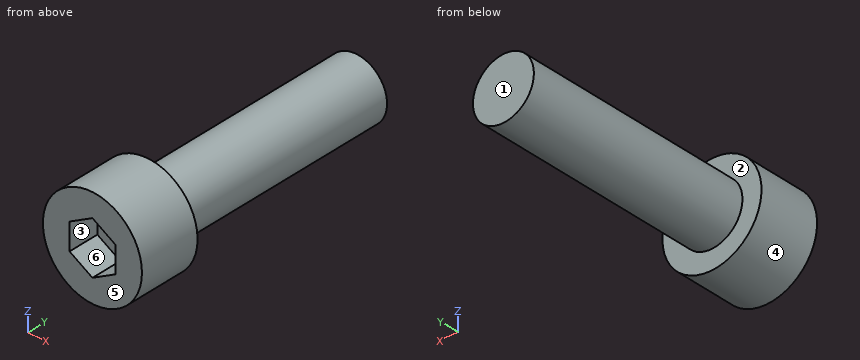
Solid Edge part; units mm, degrees
sketch "Sketch1" plane through (0, 0, 0) normal (0, -1, 0) x (1, 0, 0)
  circle A0 centre (0, 0) radius 6.5
extrude "Protrusion1" add sketch "Sketch1" against normal blind 8
sketch "Sketch2" plane through (0, 0, 0) normal (0, -1, 0) x (1, 0, 0)
  line L0 (3, 1.7321) -> (0, 3.4641)
  line L1 (0, 3.4641) -> (-3, 1.7321)
  line L2 (-3, 1.7321) -> (-3, -1.7321)
  line L3 (-3, -1.7321) -> (0, -3.4641)
  line L4 (0, -3.4641) -> (3, -1.7321)
  line L5 (3, -1.7321) -> (3, 1.7321)
extrude "ExtrudedCutout_1" cut sketch "Sketch2" against normal blind 4
sketch "Sketch3" plane through (0, 8, 0) normal (0, 1, 0) x (-1, 0, 0)
  circle A0 centre (0, 0) radius 4
extrude "ExtrudedProtrusion_2" add sketch "Sketch3" along normal blind 30
cosmetic_thread "Thread1"
properties material "Steel"
Could you check a few things on this model? Use its own coordinates, in mm. Face numbers are marked on the shaded views. A direction names the side the tool comes from. Coordinates: 2 decimals unless noted, no trailing zeros. Order: outer loops, then holes, each group sorted by start corner. A loop starts at its lowest first (then second) coordinate and runs counter-clockwise, first axis right, second up. Notation, with made-up numbers: (-16, -18) - (26, -18) arc R6 ccw to (26, -10) - close; hole circle Ø11 at (-18, 67). An arc over 180 degrees is marked (long way). Answer in a Markdown table with one row per item. Add a question column.
(1) If we section it at C-C, the plane y = 13: Please give me the cut outline in (x, z), then the cut area to 3 significant figures.
(2) If we section it at D-D, the plane z = 5.5: Please give me the cut outline in (x, y).
(3) I need wall thicknesses on L1, parallel to Y at x = -4, z = -3; L2, parallel to X at y = 18, z = -0.25; L3, parallel to Y at x = 2, z = -1.25. Which ranges of each line are inside material? Lowest first, please.
(4) If we section it at A-A, the plane z = 0: Please give me the cut outline in (x, y).
(5) Will these pins go through, and if not, where does the flat tip stop? pin 1 (4 mm diameter, centred on x = -1, y = 8.5, fed in from +Z); pin 2 (2 mm diameter, centred on x = 1.5, z = -1, fed in from -Y); pin 3 (1 mm diameter, centred on y = 20.5, z = 0, fed in from +X); pin 4 (6 mm diameter, centred on x = -3, y = 32.5, fed in from -Z).
(6) On a 3-axis mill with a long thin cutter (end or side, diameter ignored), from which of +Z, -Z, +X, -X, +Y, -Y can I reach the whole of each face in a straight line? I mean the marked faces 1, 2 and 3. Say none if no direction works.
(7) If we mould it in two halves opening along Z, with no side actions, what happens to the marked faces 4, 5 and 6? For each: released by +Z, released by -Z, zero draft, split by the parting line, or undercut.
(8) If we section it at B-B, the plane x = -1.25: Please give me the cut outline in (y, z), then the cut area to 3 significant figures.
Results are:
| question | item | result |
|---|---|---|
| 1 | outline | circle Ø8 at (0, 0) |
| 1 | area | 50.3 mm2 |
| 2 | outline | (-3.46, 0) - (3.46, 0) - (3.46, 8) - (-3.46, 8) - close |
| 3 | L1 | y = 0 to 8 |
| 3 | L2 | x = -3.99 to 3.99 |
| 3 | L3 | y = 4 to 38 |
| 4 | outline | (-6.5, 0) - (-3, 0) - (-3, 4) - (3, 4) - (3, 0) - (6.5, 0) - (6.5, 8) - (4, 8) - (4, 38) - (-4, 38) - (-4, 8) - (-6.5, 8) - close |
| 5 | pin 1 | stops at z = 6.5 |
| 5 | pin 2 | stops at y = 4 |
| 5 | pin 3 | stops at x = 4 |
| 5 | pin 4 | stops at z = -4 |
| 6 | face 1 | +Z, -Z, +X, -X, +Y |
| 6 | face 2 | +Y |
| 6 | face 3 | -Y |
| 7 | face 4 | split by the parting line |
| 7 | face 5 | zero draft |
| 7 | face 6 | undercut |
| 8 | outline | (0, -6.38) - (8, -6.38) - (8, -3.8) - (38, -3.8) - (38, 3.8) - (8, 3.8) - (8, 6.38) - (0, 6.38) - (0, 2.74) - (4, 2.74) - (4, -2.74) - (0, -2.74) - close |
| 8 | area | 308 mm2 |
